```python
from build123d import *

# Parameters (mm, degrees)
SKETCH1_W             = 40
SKETCH1_H             = 280
EXTRUDE1_DEPTH        = 16
EXTRUDE2_REACH        = 282
SKETCH2_W             = 30
SKETCH2_H             = 2.5
M4_TAPPED_HOLE1_D     = 3.3
M6_TAPPED_HOLE1_D     = 5
M5_TAPPED_HOLE1_D     = 4.2
M5_TAPPED_HOLE1_DEPTH = 13.5


with BuildPart() as part:
    # Sketch1 → Extrude1 (new body)
    with BuildSketch(Plane.XY):
        Rectangle(SKETCH1_W, SKETCH1_H)
    extrude(amount=EXTRUDE1_DEPTH)

    # Sketch2 → Extrude2 (cut, up to next)
    with BuildSketch(Plane.XZ.offset(140), mode=Mode.PRIVATE) as extrude2_sk1:
        with Locations((-5, 14.75)):
            Rectangle(SKETCH2_W, SKETCH2_H)
    extrude2_tool1 = extrude(extrude2_sk1.sketch, amount=-EXTRUDE2_REACH, mode=Mode.PRIVATE) & part.part
    add(extrude2_tool1.solids().sort_by_distance((-5, -140, 14.75))[0], mode=Mode.SUBTRACT)

    # M4 Tapped Hole1 (through all)
    with Locations(Plane.XY.offset(13.5)):
        with Locations((2.5, -120), (2.5, -60), (2.5, 0), (2.5, 60), (2.5, 120)):
            Hole(M4_TAPPED_HOLE1_D / 2)

    # M6 Tapped Hole1 (through all)
    with Locations(Plane(origin=(0, 0, 0), x_dir=(-1, 0, 0), z_dir=(0, 0, -1))):
        with Locations((0, 105), (0, -105)):
            Hole(M6_TAPPED_HOLE1_D / 2)

    # M5 Tapped Hole1
    with Locations(Plane.XY.offset(13.5)):
        with Locations((0, 80), (0, -80)):
            Hole(M5_TAPPED_HOLE1_D / 2, depth=M5_TAPPED_HOLE1_DEPTH)


solid = part.part
```
Input: part model. Units: mm. Frame: model coordinates. A direction names the side the tool comes from. Give positions to 0.01 mm unless a question says otherwise; leave off trailing zeros. Order: outer loops, then holes, each group sorted by start corner. A loop starts at its lowest first (then second) coordinate and runs counter-clockwise, first axis right, second up. Notation, with made-up numbers: (-38.75, -16.5) - (-31.75, -16.5) arc R20 ccw to (-31.75, 16.5) - close; hole circle Ø9 at (-11.75, -31). An arc over 180 degrees is marked (long way). One line per item, written item: value.
1. Cut plane A-A, the plane y = 21.5. Output: boundary loops of the cut face in (x, z).
Determined:
outline: (-20, 0) - (20, 0) - (20, 16) - (10, 16) - (10, 13.5) - (-20, 13.5) - close
2. Reachability of faces 1 (the face through (15, 2, 16)), 2 (the face through (-5, -2, 13.5)) from +Z, -Z, +X, -X, +Y, -Y: full face, straight path, thin tool, end or side. Return the list, or none.
Determined:
face 1: +Z, +X, -X, +Y, -Y
face 2: +Z, -X, +Y, -Y
3. Pin query (flat end, axial travel): pin 1 Ø8 at (x, y) = (-15, 95.5) entering from +Z; pin 2 Ø1.2 at (y, z) = (-9.5, 15) entering from -X. Return the tip coordinate at first contact, or that it passes through.
Determined:
pin 1: z = 13.5
pin 2: x = 10
4. Line query: probe 1 along Y at (x, z) = (0, 8); probe 2 along X at (y, z) = (-120, 4); probe 3 along Z at (x, y) = (-16, 41.5). Output: solid intervals per line, ascending.
Determined:
probe 1: -140 to -107.5, -102.5 to -82.1, -77.9 to 77.9, 82.1 to 102.5, 107.5 to 140
probe 2: -20 to 0.85, 4.15 to 20
probe 3: 0 to 13.5
5. Cut plane B-B, the plane x = -12. Output: boundary loops of the cut face in (y, z), and give its area (3 significant figures).
Determined:
outline: (-140, 0) - (140, 0) - (140, 13.5) - (-140, 13.5) - close
area: 3,780 mm2
